Check sheet for the modelled part. Datum: model origin and axes. Units: mm. A direction names the side the tool comes from. Coordinates: 2 decimals unless noted, no trailing zeros. Write each loop counter-clockwise with the first axis right and the second up, starting at its lowest first coordinate (ties: lowest second). Pieces come first, ordered by that corner, then holes. Notation, with made-up numbers: M 77,1 L 84,1 A30 ccw 84,27 Z; hole C -32,-1.5 d10. An arc over 180 degrees is marked long. Answer as CSV lines item,"result".
Autodesk Inventor part; units mm, degrees
ref_plane "YZ Plane" through (0, 0, 0) normal (1, 0, 0) x (0, 1, 0)
ref_plane "XZ Plane" through (0, 0, 0) normal (0, 1, 0) x (-1, 0, 0)
ref_plane "XY Plane" through (0, 0, 0) normal (0, 0, 1) x (1, 0, 0)
sketch "Sketch1" plane through (0, 0, 0) normal (0, 0, 1) x (1, 0, 0)
  line L0 (14.1854, 26.7901) -> (14.1854, -123.2099)
  line L1 (14.1854, -123.2099) -> (39.1854, -123.2099)
  line L2 (39.1854, -123.2099) -> (39.1854, 26.7901)
  line L3 (39.1854, 26.7901) -> (14.1854, 26.7901)
  circle A0 centre (26.6854, 10.2901) radius 9.5
  circle A1 centre (26.6854, -48.2099) radius 6
  circle A2 centre (37.1854, -8.2099) radius 3
  line L4 (39.1854, -5.2099) -> (14.1854, -5.2099)
  line L5 (39.1854, -11.2099) -> (14.1854, -11.2099)
  circle A3 centre (26.6854, 23.2901) radius 1.5
  line L6 (26.6854, 19.7901) -> (20.6854, 19.7901)
  line L7 (26.6854, 21.7901) -> (21.9472, 21.7901)
  line L8 (26.6854, 24.7901) -> (23.6854, 24.7901)
  line L9 (26.6854, 10.2901) -> (21.9472, 10.2901)
  circle A4 centre (26.6854, -2.7099) radius 1.5
  line L10 (14.1854, -48.2099) -> (17.1854, -48.2099)
  circle A5 centre (26.6854, -106.7099) radius 9.5
  circle A6 centre (37.1854, -88.2099) radius 3
  line L11 (39.1854, -91.2099) -> (14.1854, -91.2099)
  line L12 (39.1854, -85.2099) -> (14.1854, -85.2099)
  circle A7 centre (26.6854, -119.7099) radius 1.5
  line L13 (26.6854, -116.2099) -> (20.6854, -116.2099)
  line L14 (26.6854, -118.2099) -> (21.9472, -118.2099)
  line L15 (26.6854, -121.2099) -> (23.6854, -121.2099)
  line L16 (26.6854, -106.7099) -> (21.9472, -106.7099)
  circle A8 centre (26.6854, -93.7099) radius 1.5
  dimension "d0" = 150
  dimension "d1" = 25
  dimension "d6" = 12.5
  dimension "d8" = 12
  dimension "d12" = 75
  dimension "d13" = 6
  dimension "d33" = 3
  dimension "d81" = 3.5
  dimension "d83" = 2
  dimension "d84" = 2
  dimension "d85" = 16.5
  dimension "d130" = 12.5
  dimension "d131" = 12.5
extrude "Extrusion1" add sketch "Sketch1" along normal blind 70 contours L3 L2 L4 L0 | L4 A2 L5 L0 | L5 L2 L12 L0 | L4 L2 A2 | A2 L2 | A2 L2 L5 | L12 A6 L11 L0 | L11 L2 L1 L0 | L12 L2 A6 | A6 L2 | A6 L2 L11 | A3 | A4 | A7 | A8 picked at (35.982, -7.4645) picked at (36.2539, -87.8584)
sketch "Sketch2" plane through (39.1854, -123.2099, 0) normal (1, 0, 0) x (0, 0, -1)
  circle A0 centre (-27.5, 100) radius 3
  circle A1 centre (-42.5, 100) radius 3
  circle A2 centre (-55, 120) radius 3
  circle A3 centre (-15, 120) radius 3
  line L0 (0, 150) -> (-70, 150)
  line L1 (0, 0) -> (0, 150)
  line L2 (-70, 0) -> (-70, 150)
  line L3 (0, 75) -> (-12, 75)
  circle A4 centre (-27.5, 50) radius 3
  circle A5 centre (-42.5, 50) radius 3
  circle A6 centre (-55, 30) radius 3
  circle A7 centre (-15, 30) radius 3
  dimension "d17" = 6
  dimension "d18" = 6
  dimension "d19" = 6
  dimension "d20" = 6
  dimension "d21" = 30
  dimension "d24" = 30
  dimension "d25" = 15
  dimension "d26" = 15
  dimension "d204" = 50
  dimension "d205" = 50
  dimension "d206" = 12.5
  dimension "d207" = 12.5
sketch "Sketch5" plane through (0, 0, 0) normal (0, 0, -1) x (-1, 0, 0)
  circle A0 centre (-26.6854, 22.2901) radius 1.5
  line L0 (-39.1854, 26.7901) -> (-14.1854, 26.7901)
  circle A1 centre (-26.6854, 10.2901) radius 9.5
  line L1 (-14.1854, 26.7901) -> (-14.1854, -123.2099)
  circle A2 centre (-26.6854, -1.7099) radius 1.5
  line L2 (-14.1854, 26.7901) -> (-14.1854, -123.2099)
  line L3 (-14.1854, -48.2099) -> (-19.6815, -48.2099)
  circle A3 centre (-26.6854, -118.7099) radius 1.5
  circle A4 centre (-26.6854, -94.7099) radius 1.5
  circle A5 centre (-26.6854, 10.2901) radius 9.5
  line L4 (-26.6854, 0.7901) -> (-19.8619, 0.7901)
  dimension "d53" = 3
  dimension "d55" = 12.5
  dimension "d56" = 3
  dimension "d58" = 12.5
  dimension "d79" = 12
  dimension "d199" = 12
sketch "Sketch7" plane through (0, 0, 70) normal (0, 0, 1) x (1, 0, 0)
  circle A0 centre (26.6854, 22.2901) radius 1.5
  line L0 (39.1854, 26.7901) -> (14.1854, 26.7901)
  line L1 (39.1854, -123.2099) -> (39.1854, 26.7901)
  circle A1 centre (26.6854, -1.7099) radius 1.5
  line L2 (39.1854, -48.2099) -> (34.5459, -48.2099)
  circle A2 centre (26.6854, -118.7099) radius 1.5
  line L3 (39.1854, -123.2099) -> (14.1854, -123.2099)
  line L4 (39.1854, 26.7901) -> (39.1854, -123.2099)
  line L5 (26.6854, -106.7099) -> (25.3096, -106.7099)
  circle A3 centre (26.6854, -94.7099) radius 1.5
  circle A4 centre (26.6854, 10.2901) radius 9.5
  dimension "d87" = 3
  dimension "d89" = 12.5
thread "Thread16"
sketch "Sketch8" plane through (0, 0, 0) normal (0, 0, -1) x (-1, 0, 0)
  line L0 (-39.1854, -48.2099) -> (-26.6854, -48.2099)
  circle A0 centre (-26.6854, -48.2099) radius 11
  circle A1 centre (-26.6854, -48.2099) radius 6
  point P0 (0, 0)
  dimension "d113" = 12.5
  dimension "d114" = 22
extrude "Extrusion9" cut sketch "Sketch8" against normal blind 10
sketch "Sketch9" plane through (0, 0, 0) normal (0, 0, -1) x (-1, 0, 0)
  circle A0 centre (-26.6854, -48.2099) radius 11
  circle A1 centre (-26.6854, -48.2099) radius 11
  circle A2 centre (-26.6854, -34.2099) radius 1.5
  circle A3 centre (-26.6854, -62.2099) radius 1.5
  line L0 (-39.1854, -123.2099) -> (-39.1854, 26.7901)
  line L1 (-14.1854, 26.7901) -> (-14.1854, -123.2099)
  dimension "d117" = 22
  dimension "d118" = 3
  dimension "d119" = 3
  dimension "d120" = 14
  dimension "d121" = 14
  dimension "d122" = 12.5
  dimension "d123" = 12.5
hole "Agujero1" at (39.1854, -3.2099, 55) at (39.1854, -23.2099, 42.5) at (39.1854, -23.2099, 27.5) at (39.1854, -3.2099, 15) at (39.1854, -93.2099, 55) at (39.1854, -73.2099, 42.5) at (39.1854, -73.2099, 27.5) at (39.1854, -93.2099, 15) direction (-1, 0, 0) diameter 6 depth 20 tip angle 118
hole "Agujero2" at (26.6854, -1.7099, 0) at (26.6854, 22.2901, 0) at (26.6854, -94.7099, 0) at (26.6854, -118.7099, 0) direction (0, 0, 1) diameter 3 depth 5 tip angle 118
thread "Rosca21"
thread "Rosca22"
thread "Rosca23"
thread "Rosca24"
hole "Agujero3" at (26.6854, 22.2901, 70) at (26.6854, -1.7099, 70) at (26.6854, -94.7099, 70) at (26.6854, -118.7099, 70) direction (0, 0, -1) diameter 3 depth 5 tip angle 118
thread "Rosca25"
thread "Rosca26"
thread "Rosca27"
thread "Rosca28"
hole "Agujero4" at (26.6854, -34.2099, 0) at (26.6854, -62.2099, 0) direction (0, 0, 1) diameter 3 depth 8 tip angle 118
thread "Rosca29"
thread "Rosca30"
sketch "Boceto10" plane through (0, 0, 70) normal (0, 0, 1) x (1, 0, 0)
  circle A0 centre (26.6854, -48.2099) radius 6
  circle A1 centre (26.6854, -48.2099) radius 7
  point P0 (0, 0)
  dimension "d184" = 14
hole "Agujero5" at (26.6854, -48.2099, 70) direction (0, 0, -1) diameter 14 depth 0.01 tip angle 118
sketch "Boceto11" plane through (14.1854, -123.2099, 0) normal (0, -1, 0) x (1, 0, 0)
  line L0 (6.5, 69.3891) -> (6.5, 10)
  circle A0 centre (3, 31) radius 1.5
  circle A1 centre (3, 39) radius 1.5
  line L1 (0, 0) -> (0, 70)
  line L2 (0, 70) -> (25, 70)
  point P0 (-14.1854, 0)
  dimension "d209" = 3
  dimension "d210" = 3
  dimension "d211" = 3
  dimension "d212" = 31
  dimension "d213" = 3
  dimension "d214" = 8
hole "Agujero7" at (17.1854, -123.2099, 31) at (17.1854, -123.2099, 39) direction (0, 1, 0) diameter 3 depth 10 tip angle 118
thread "Thread31"
thread "Thread32"
thread "Rosca33"
thread "Rosca34"
thread "Rosca35"
thread "Rosca36"
thread "Rosca37"
thread "Rosca38"
thread "Rosca39"
thread "Rosca40"
equation "\"d211\" = d213"
properties part number "Bloque - Vinculo Cabezal" material "Aluminum 6061"
1) Thickness scan on line 1 along Z through (x, y) = (34.75, -23); line 2 along Y through (x, z) = (30.5, 49.5); line 3 along Y through (x, z) = (32.5, 3). Record the ranges inside material, lowest first.
Answer key:
line 1,"z = 0 to 24.51, 30.49 to 39.51, 45.49 to 70"
line 2,"y = -123.21 to -115.41, -98.01 to -52.84, -43.58 to 1.59, 18.99 to 26.79"
line 3,"y = -123.21 to -114.22, -99.2 to -57.55, -38.87 to 2.78, 17.8 to 26.79"
2) Mould release check, pull along X, two halves, no side actions. Record for faces 6 (the face through (29, -3.3, 18)), 7 (the face through (14.185, -47, 35)), 8 (the face through (20.772, -38.935, 4.93)): pulls with the +X half, pulls with the -X half, needs draft (parallel to the pull), parting line crosses it, or undercut.
Answer key:
face 6,"needs draft"
face 7,"pulls with the -X half"
face 8,"undercut"
3) Section check A-A, the plane z = 60. Record the boundary of the cut face in (x, y), plus the area to 3 significant figures.
Answer key:
outline,"M 14.19,-123.21 L 39.19,-123.21 L 39.19,26.79 L 14.19,26.79 Z; hole C 26.69,-106.71 d19; hole C 26.69,10.29 d19; hole C 26.69,-48.21 d12"
area,"3,070 mm2"
4) Depth check by flat-ended pin: P1, Ø5.5, axis at y = -23.21, z = 42.5, coming from the +X side; P2, Ø1.5, axis at x = 33.5, y = -27, coming from the -Z side; P3, Ø13, axis at x = 26.69, y = -48.21, coming from the -Z side; P4, Ø3.5, axis at y = -93.21, z = 55, coming from the +X side. Enter the tip coordinate at first touch or a pass-through.
Answer key:
P1,"stops at x = 19.04"
P2,"stops at z = 0"
P3,"stops at z = 10"
P4,"stops at x = 18.43"
5) Section check B-B, the plane x = 23.5. Give the number of separate pieces and of enclosed holes in the cut face, plus the area to 3 significant figures.
Answer key:
separate pieces,"4"
enclosed holes,"8"
area,"6,950 mm2"
6) Tool access check on faces 1 (the face through (26.62, -117.21, 67.46)), 2 (the face through (29.05, -95.24, 57.21)), 3 (the face through (39.185, -49, 35)), 4 (the face through (16.172, -118.14, 32.106)), 5 (the face through (25.672, -119.815, 2.535)). Record the directions out of +Z, -Z, +X, -X, +Y, -Y that give a thin tool (end or side, any length) a straight path to the whole face; none if there is none.
Answer key:
face 1,"+Z"
face 2,"+X"
face 3,"+Z, -Z, +X, +Y, -Y"
face 4,"-Y"
face 5,"-Z"
